```python
from build123d import *

# Parameters (mm, degrees)
SKETCH1_R           = 82.55
SKETCH1_R_2         = 76.55
BOSS_EXTRUDE1_DEPTH = 380
SKETCH2_R           = 80.55
CUT_EXTRUDE1_DEPTH  = 170
SKETCH3_R           = 80.55
CUT_EXTRUDE2_DEPTH  = 155


with BuildPart() as part:
    # Sketch1 → Boss-Extrude1 (new body)
    with BuildSketch(Plane(origin=(0, 0, 0), x_dir=(1, 0, 0), z_dir=(0, 1, 0))):
        Circle(SKETCH1_R)
        Circle(SKETCH1_R_2, mode=Mode.SUBTRACT)
    extrude(amount=BOSS_EXTRUDE1_DEPTH)

    # Sketch2 → Cut-Extrude1 (cut)
    with BuildSketch(Plane.XZ):
        Circle(SKETCH2_R)
    extrude(amount=-CUT_EXTRUDE1_DEPTH, mode=Mode.SUBTRACT)

    # Sketch3 → Cut-Extrude2 (cut)
    with BuildSketch(Plane(origin=(0, 380, 0), x_dir=(1, 0, 0), z_dir=(0, 1, 0))):
        Circle(SKETCH3_R)
    extrude(amount=-CUT_EXTRUDE2_DEPTH, mode=Mode.SUBTRACT)


solid = part.part
```
Can you work these out from the model? Positions are in its coordinate system, mm. A direction names the side the tool comes from. Round coordinates to 2 decimals unless told otherwise and drop trailing zeros. Loops run counter-clockwise (first coordinate to the right, second up) from the corner with the lowest first, then second, coordinate; pieces in that order, holes last. Notation, with made-up numbers: (78.5, 19) -> (128.5, 19) arc R17 cw to (128.5, 43) -> close; hole circle Ø3 at (16.5, -26). An arc over 180 degrees is marked (long way). Answer in a Markdown table with one row per item.
Item 1: If I drill on probe 1 along X at (y, z) = (328.5, 0); probe 2 along Z at (x, y) = (-29, 254.5); probe 3 along Z at (x, y) = (-1.5, 93), over which ranges is the centre line in solid material (lowest first)?
Answer block:
| item | result |
|---|---|
| probe 1 | -82.55 to -80.55, 80.55 to 82.55 |
| probe 2 | -77.29 to -75.15, 75.15 to 77.29 |
| probe 3 | -82.54 to -80.54, 80.54 to 82.54 |
Item 2: On a 3-axis mill with a long thin cutter (end or side, diameter ignored), from which of +Z, -Z, +X, -X, +Y, -Y can I reach the whole of each face in a straight line? I mean faces 1 (the flat face through (18, 0, 79)), 2 (the cylindrical face through (76.83, 303.59, -24.2)), 3 (the cylindrical face through (76.83, 83.81, 24.2)). Say none if no direction works.
Answer block:
| item | result |
|---|---|
| face 1 | +Z, -Z, +X, -X, -Y |
| face 2 | +Y |
| face 3 | -Y |
Item 3: Suppose I cut it at C-C, the plane y = 267. List the corners of the cut face in (x, z) for me, plus the area to 3 significant figures.
Answer block:
| item | result |
|---|---|
| outline | circle Ø165.1 at (0, 0); hole circle Ø161.1 at (0, 0) |
| area | 1,020 mm² |
Item 4: We'd pull the mould along X, two halves only. Please class faces 4 (the flat face through (18, 380, 79)), 5 (the cylindrical face through (-9.965, 197.115, -75.899)), 6 (the cylindrical face through (-17.895, 187.34, 80.587)): released by +X, released by -X, zero draft, split by the parting line, or undercut.
Answer block:
| item | result |
|---|---|
| face 4 | zero draft |
| face 5 | undercut |
| face 6 | split by the parting line |
Item 5: Will these pins go through, and if not, where does the flat tip stop? P1, Ø1, axis at x = 53.5, y = 284, coming from the +Z side; P2, Ø4, axis at y = 268, z = 9, coming from the +X side; P3, Ø5, axis at x = 4, y = 329, coming from the +Z side.
Answer block:
| item | result |
|---|---|
| P1 | z = 63.29 |
| P2 | x = 82.25 |
| P3 | z = 82.54 |
Item 6: Suppose I cut it at B-B, the plane x = 0. List the corners of the cut face in (y, z) for me.
Answer block:
| item | result |
|---|---|
| outline | (0, -82.55) -> (380, -82.55) -> (380, -80.55) -> (225, -80.55) -> (225, -76.55) -> (170, -76.55) -> (170, -80.55) -> (0, -80.55) -> close; (0, 80.55) -> (170, 80.55) -> (170, 76.55) -> (225, 76.55) -> (225, 80.55) -> (380, 80.55) -> (380, 82.55) -> (0, 82.55) -> close |
Item 7: Suppose I cut it at A-A, the plane z = 0. List the corners of the cut face in (x, y) for me.
Answer block:
| item | result |
|---|---|
| outline | (-82.55, 0) -> (-80.55, 0) -> (-80.55, 170) -> (-76.55, 170) -> (-76.55, 225) -> (-80.55, 225) -> (-80.55, 380) -> (-82.55, 380) -> close; (76.55, 170) -> (80.55, 170) -> (80.55, 0) -> (82.55, 0) -> (82.55, 380) -> (80.55, 380) -> (80.55, 225) -> (76.55, 225) -> close |
